Geometry: final body of the model. Coordinates: model frame, mm. Round coordinates to 2 decimals unless told otherwise and drop trailing zeros. Loops run counter-clockwise (first coordinate to the right, second up) from the corner with the lowest first, then second, coordinate; pieces in that order, holes last. Notation, with made-up numbers: (-13.5, -10) - (40.5, -10) arc R25 ccw to (40.5, 23) - close; hole circle Ø11 at (39, -10). An arc over 180 degrees is marked (long way). Use CSV: the item, a comma, the result in double quotes.
from build123d import *

# Parameters (mm, degrees)
F0_R     = 114.3
F1_DEPTH = 25.4
F2_DEPTH = 12.7
F3_DEPTH = 6.35
F4_W     = 57.15
F4_H     = 57.15
F5_DEPTH = 2.54
F6_W     = 12.7
F6_H     = 1.27
F7_DEPTH = 1.27


with BuildPart() as f1:
    # F0 (on Front) → F1 (new body)
    with BuildSketch(Plane.XZ):
        Circle(F0_R)
    extrude(amount=F1_DEPTH)

    # F2 (cut): a face of the model
    f2_faces = [f1.faces().sort_by_distance(p)[0] for p in [
        (0, -25.4, 0),
    ]]
    extrude(f2_faces, amount=-F2_DEPTH, mode=Mode.SUBTRACT)

    # F3 (cut): a face of the model
    f3_faces = [f1.faces().sort_by_distance(p)[0] for p in [
        (0, -12.7, 0),
    ]]
    extrude(f3_faces, amount=-F3_DEPTH, mode=Mode.SUBTRACT)

    # F4 (on face) → F5 (cut)
    with BuildSketch(Plane(origin=(0, 0, 0), x_dir=(-1, 0, 0), z_dir=(0, 1, 0))):
        Rectangle(F4_W, F4_H)
    extrude(amount=-F5_DEPTH, mode=Mode.SUBTRACT)

    # F6 (on face) → F7 (cut)
    with BuildSketch(Plane(origin=(0, 0, 0), x_dir=(-1, 0, 0), z_dir=(0, 1, 0))):
        with Locations((0, 100.2205033398)):
            Rectangle(F6_W, F6_H)
    extrude(amount=-F7_DEPTH, mode=Mode.SUBTRACT)


solid = f1.part
Item 1: Section B-B on z = 0. Return the cut outline in (x, y) (3 decimals), plus the area to 3 significant figures.
Final values:
outline,"(-114.3, -6.35) - (114.3, -6.35) - (114.3, 0) - (28.575, 0) - (28.575, -2.54) - (-28.575, -2.54) - (-28.575, 0) - (-114.3, 0) - close"
area,"1,310 mm²"
Item 2: Material intervals for line 1 (X direction, y = -1, z = -1) (3 decimals); line 2 (Y direction, x = -20.5, z = 23); line 3 (X direction, y = -5, z = -3), sorted ascending.
Final values:
line 1,"x = -114.296 to -28.575, 28.575 to 114.296"
line 2,"y = -6.35 to -2.54"
line 3,"x = -114.26 to 114.26"
Item 3: Section D-D on z = 87. Return the cut outline in (x, y), plus the area to 3 significant figures.
Final values:
outline,"(-74.13, -6.35) - (74.13, -6.35) - (74.13, 0) - (-74.13, 0) - close"
area,"941 mm²"
Item 4: Mould query, pull axis Z, two halves, no side actions, for faces 1 (the flat face through (-2, -6.35, 2)), 2 (the cylindrical face through (-114.19, -3.13, 5.03)), 3 (the flat face through (0, -2.54, 0)). Classes: released by +Z, released by -Z, zero draft, split by the parting line, or undercut.
Final values:
face 1,"zero draft"
face 2,"split by the parting line"
face 3,"undercut"
Item 5: Pin query (flat end, axial travel): P1, Ø3, axis at x = 13, y = -1.5, coming from the -Z side; P2, Ø1, axis at x = -2, z = 100, coming from the +Y side; P3, Ø1, axis at x = -36, y = -5, coming from the +Z side; P4, Ø0.8, axis at y = -2, z = -4, coming from the +X side. Return the tip coordinate at first contact, or that it passes through.
Final values:
P1,"stops at z = -113.72"
P2,"stops at y = 0"
P3,"stops at z = 108.65"
P4,"stops at x = 114.24"
Item 6: Section C-C on y = -4.5. Return the cut outline in (x, z), plus the area to 3 significant figures.
Final values:
outline,"circle Ø228.6 at (0, 0)"
area,"41,000 mm²"
